Part model, mm, in its own coordinate system. Face numbers are marked on the shaded views. A direction names the side the tool comes from. Give positions to 0.01 mm unless a question says otherwise; leave off trailing zeros.
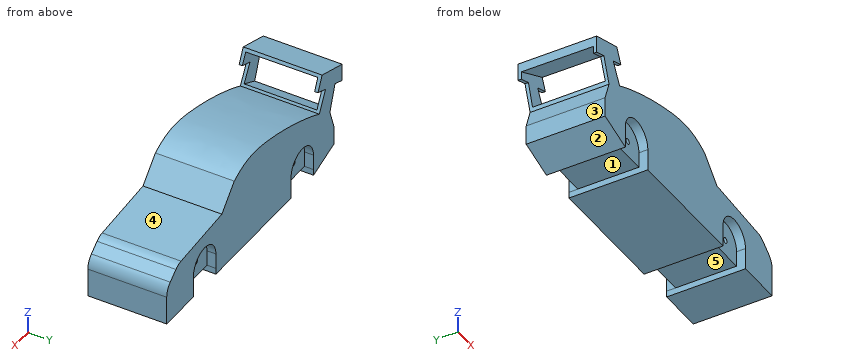
```python
from build123d import *

# Parameters (mm, degrees)
F1_DEPTH  = 38.1
F3_DEPTH  = 25.4
F6_DEPTH  = 4.318
F8_DEPTH  = 4.318
F9_R      = 1.3609782851
F9_R_2    = 1.3503546706
F10_DEPTH = 61.214


# Not quite as in the source:
# - a feature names something its author has since deleted; it is built from what else it names


with BuildPart() as f1:
    # F0 (on Front) → F1 (new body)
    with BuildSketch(Plane.XZ):
        with BuildLine():
            Line((52.0340008008, 9.3591057662), (47.4384056476, 12.9927370075))
            ThreePointArc((47.4384056476, 12.9927370075), (45.4749605723, 14.1169814212), (43.2679541409, 14.615142718))
            Line((43.2679541409, 14.615142718), (10.0584002212, 17.5260007381))
            Line((10.0584002212, 17.5260007381), (0, 28.1940009445))
            add(Edge.make_bspline(
                [(0, 28.1940009445), (-9.1002955269, 33.2901659502), (-24.9064630473, 33.5549116559), (-55.7131559047, 24.6859865442), (-69.1292500573, 18.2258343206)],
                knots=[0, 0, 0, 0, 0.4163863711, 0.8919338321, 0.8919338321, 0.8919338321, 0.8919338321], degree=3))
            add(Edge.make_bspline(
                [(-69.1292500573, 18.2258343206), (-72.1780012369, 16.7577917973), (-75.0713687219, 15.2003305751), (-77.7240023017, 13.5635994375)],
                knots=[0.8919338321, 0.8919338321, 0.8919338321, 0.8919338321, 1, 1, 1, 1], degree=3))
            Line((-77.7240023017, 13.5635994375), (-80.9243991971, 4.4677392631))
            Line((-80.9243991971, 4.4677392631), (-80.9243991971, -5.0292001106))
            Line((-80.9243991971, -5.0292001106), (-64.465200973, -10.5156))
            Line((-64.465200973, -10.5156), (-64.465200973, -7.498764433))
            Line((-64.465200973, -7.498764433), (-64.465200973, 0))
            ThreePointArc((-64.465200973, 0), (-55.321200973, 9.144), (-46.177200973, 0))
            Line((-46.177200973, 0), (-46.177200973, -7.498764433))
            Line((-46.177200973, -7.498764433), (-46.177200973, -10.5156))
            Line((-46.177200973, -10.5156), (14.9299539626, -10.5156))
            Line((14.9299539626, -10.5156), (14.9299539626, -7.498764433))
            Line((14.9299539626, -7.498764433), (14.9299539626, 0))
            ThreePointArc((14.9299539626, 0), (24.076577276, 9.1466233134), (33.2232005894, 0))
            Line((33.2232005894, 0), (33.2232005894, -7.498764433))
            Line((33.2232005894, -7.498764433), (33.2232005894, -10.5156004429))
            Line((33.2232005894, -10.5156004429), (54.9278818071, -10.5156004429))
            Line((54.9278818071, -10.5156004429), (54.9278818071, 3.3817987423))
            ThreePointArc((54.9278818071, 3.3817987423), (54.1663592887, 6.7022936804), (52.0340008008, 9.3591057662))
        make_face()
        with BuildLine():
            add(Edge.make_bspline(
                [(-69.1292500573, 18.2258343206), (-72.1780012369, 16.7577917973), (-75.0713687219, 15.2003305751), (-77.7240023017, 13.5635994375)],
                knots=[0.8919338321, 0.8919338321, 0.8919338321, 0.8919338321, 1, 1, 1, 1], degree=3))
            Line((-69.1292500573, 18.2258343206), (-74.2949992421, 27.8891995555))
            Line((-74.2949992421, 27.8891995555), (-81.9149985909, 25.7555991411))
            Line((-81.9149985909, 25.7555991411), (-77.7240023017, 13.5635994375))
        make_face()
        with BuildLine():
            Line((14.9299539626, -7.498764433), (33.2232005894, -7.498764433))
            Line((33.2232005894, -7.498764433), (33.2232005894, 0))
            ThreePointArc((33.2232005894, 0), (24.076577276, 9.1466233134), (14.9299539626, 0))
            Line((14.9299539626, 0), (14.9299539626, -7.498764433))
        make_face()
        Polygon((-81.9149985909, 25.7555991411), (-74.2949992421, 27.8891995555), (-68.0850669491, 30.023861943), (-71.4375004172, 37.033200264), (-87.724568169, 32.1564003825), (-87.724568169, 23.7585613183), align=None)
        with BuildLine():
            Line((-64.465200973, -7.498764433), (-46.177200973, -7.498764433))
            Line((-46.177200973, -7.498764433), (-46.177200973, 0))
            ThreePointArc((-46.177200973, 0), (-55.321200973, 9.144), (-64.465200973, 0))
            Line((-64.465200973, 0), (-64.465200973, -7.498764433))
        make_face()
    extrude(amount=F1_DEPTH)

    # F2 (on face) → F3 (cut)
    with BuildSketch(Plane(origin=(-43.723380858, 0, -20.9120631104), x_dir=(0, 1, 0), z_dir=(0.9021271467, 0, 0.4314702901))):
        Polygon((-36.6774983704, 47.6490445435), (-1.5018450795, 47.5782938302), (-1.6934617888, 62.6805573702), (-36.4830493927, 62.532402575), align=None)
    extrude(amount=-F3_DEPTH, mode=Mode.SUBTRACT)

    # F5 (on face) → F6 (cut)
    with BuildSketch(Plane.XZ.offset(38.1)):
        with BuildLine():
            Line((-64.465200973, 0), (-64.465200973, -7.498764433))
            Line((-64.465200973, -7.498764433), (-46.177200973, -7.498764433))
            Line((-46.177200973, -7.498764433), (-46.177200973, 0))
            ThreePointArc((-46.177200973, 0), (-55.321200973, 9.144), (-64.465200973, 0))
        make_face()
        with BuildLine():
            Line((14.9299539626, 0), (14.9299539626, -7.498764433))
            Line((14.9299539626, -7.498764433), (33.2232005894, -7.498764433))
            Line((33.2232005894, -7.498764433), (33.2232005894, 0))
            ThreePointArc((33.2232005894, 0), (24.076577276, 9.1466233134), (14.9299539626, 0))
        make_face()
    extrude(amount=-F6_DEPTH, mode=Mode.SUBTRACT)

    # F7 (on face) → F8 (cut)
    with BuildSketch(Plane.XZ):
        with BuildLine():
            Line((14.9592272937, -8.4022274241), (33.2223922014, -8.4022274241))
            Line((33.2223922014, -8.4022274241), (33.2223922014, 0))
            ThreePointArc((33.2223922014, 0), (24.0908097476, 9.1315824538), (14.9592272937, 0))
            Line((14.9592272937, 0), (14.9592272937, -8.4022274241))
        make_face()
        with BuildLine():
            Line((-64.3822327256, -7.5330701657), (-46.1474433541, -7.5330701657))
            Line((-46.1474433541, -7.5330701657), (-46.1474433541, 0))
            ThreePointArc((-46.1474433541, 0), (-55.2648380399, 9.1173946857), (-64.3822327256, 0))
            Line((-64.3822327256, 0), (-64.3822327256, -7.5330701657))
        make_face()
    extrude(amount=F8_DEPTH, mode=Mode.SUBTRACT)

    # F9 (on face) → F10 (cut)
    with BuildSketch(Plane.XZ.offset(33.782)):
        with Locations((-55.321200973, 0)):
            Circle(F9_R)
        with Locations((24.0739539626, 0)):
            Circle(F9_R_2)
    extrude(amount=-F10_DEPTH, mode=Mode.SUBTRACT)


solid = f1.part
```
1) 3-axis set-ups, long thin cutter, end or side, ignore diameter. For the marked faces 1 and 2: which of +Z, -Z, +X, -X, +Y, -Y reach the whole face in a straight line?
Answers follow:
face 1: -Z, +Y, -Y
face 2: -Z, -X, +Y, -Y
2) Saw through at A-A, the plane y = -11. Count the separate pieces of the cut face and the enclosed holes in it, then the cut area to 3 significant figures.
Answers follow:
separate pieces: 2
enclosed holes: 2
area: 4,340 mm2
3) Wall check: L1, parallel to Y at x = -81, z = 29.5; L2, parallel to Z at x = -76, y = -25.5; L3, parallel to Z at x = -31.5, y = -25.5. Give the ranges that are in metal, low to high.
Answers follow:
L1: y = -38.1 to -36.5, -1.68 to 0
L2: z = -6.67 to 16.44, 33.02 to 35.67
L3: z = -10.52 to 30.71
4) Two-plate mould, pull along X, no slides. Class the marked faces 3, 4 and 5: +X half, -X half, draft (parallel to the pull), parting line (faces both ways), or undercut.
Answers follow:
face 3: -X half
face 4: +X half
face 5: undercut
5) Pin check, flat tips, straight feed: pin 1 Ø5 at (x, z) = (-58.5, 3.5) entering from +Y; pin 2 Ø4.5 at (y, z) = (-13, 1) entering from -X; pin 3 Ø2 at (y, z) = (-14, 17) entering from -X; pin 4 Ø2.5 at (x, z) = (24.07, 0) entering from -Y. Stop position of each tip, or through.
Answers follow:
pin 1: stops at y = -4.32
pin 2: stops at x = -80.92
pin 3: stops at x = -76.88
pin 4: passes through
